Geometry check sheet. Reference: drawing and pictorial views, mm from the part's lowest x, y, z. Coordinates: 2 decimals unless noted, no trailing zeros. Write each loop counter-clockwise with the first axis right and the second up, starting at its lowest first coordinate (ties: lowest second). Pieces come first, ordered by that corner, then holes. Notation, with made-up numbers: (45.5, 76.5) - (57.5, 76.5) arc R13 cw to (57.5, 82.5) - close; hole circle Ø5 at (-13, 38). An arc over 180 degrees is marked (long way). Use one line per item in the form item = value. Start each with the question number.
(1) Material ranges on line 1 (Z direction, x = 19, y = 1.65); line 2 (X direction, y = 3.65, z = 2.5); line 3 (Z direction, x = 80, y = 3.85), recorded low to high. Write a range as [from, to].
(2) Sectioned sample at C-C (x = 119). Record the cut outline in (y, z).
(3) Sectioned sample at A-A (x = 69.6). Record the cut outline in (y, z), and give its area (3 significant figures).
(4) Sectioned sample at D-D (z = 2). Record the cut outline in (x, y).
(5) Sectioned sample at B-B (y = 2). Count the separate pieces of the cut face and the enclosed holes in it, and give its area (3 significant figures).
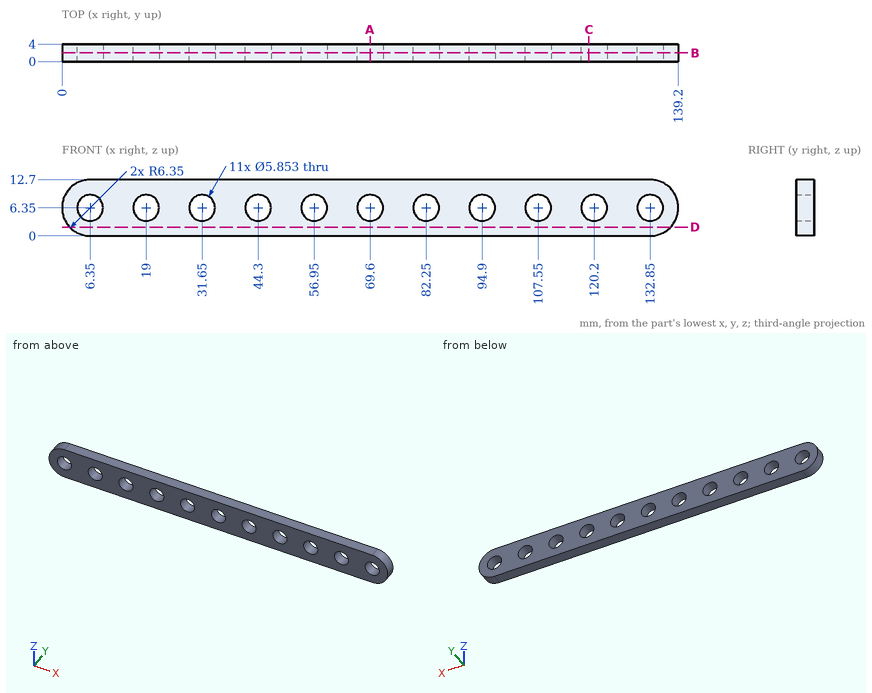
Answers below:
q1.line_1 = [0, 3.42], [9.28, 12.7]
q1.line_2 = [1.3, 137.9]
q1.line_3 = [0, 4.48], [8.22, 12.7]
q2.outline = (0, 0) - (4, 0) - (4, 3.68) - (0, 3.68) - close; (0, 9.02) - (4, 9.02) - (4, 12.7) - (0, 12.7) - close
q3.outline = (0, 0) - (4, 0) - (4, 3.42) - (0, 3.42) - close; (0, 9.28) - (4, 9.28) - (4, 12.7) - (0, 12.7) - close
q3.area = 27.4 mm2
q4.outline = (1.72, 0) - (137.48, 0) - (137.48, 4) - (1.72, 4) - close
q5.separate_pieces = 1
q5.enclosed_holes = 11
q5.area = 1,440 mm2
